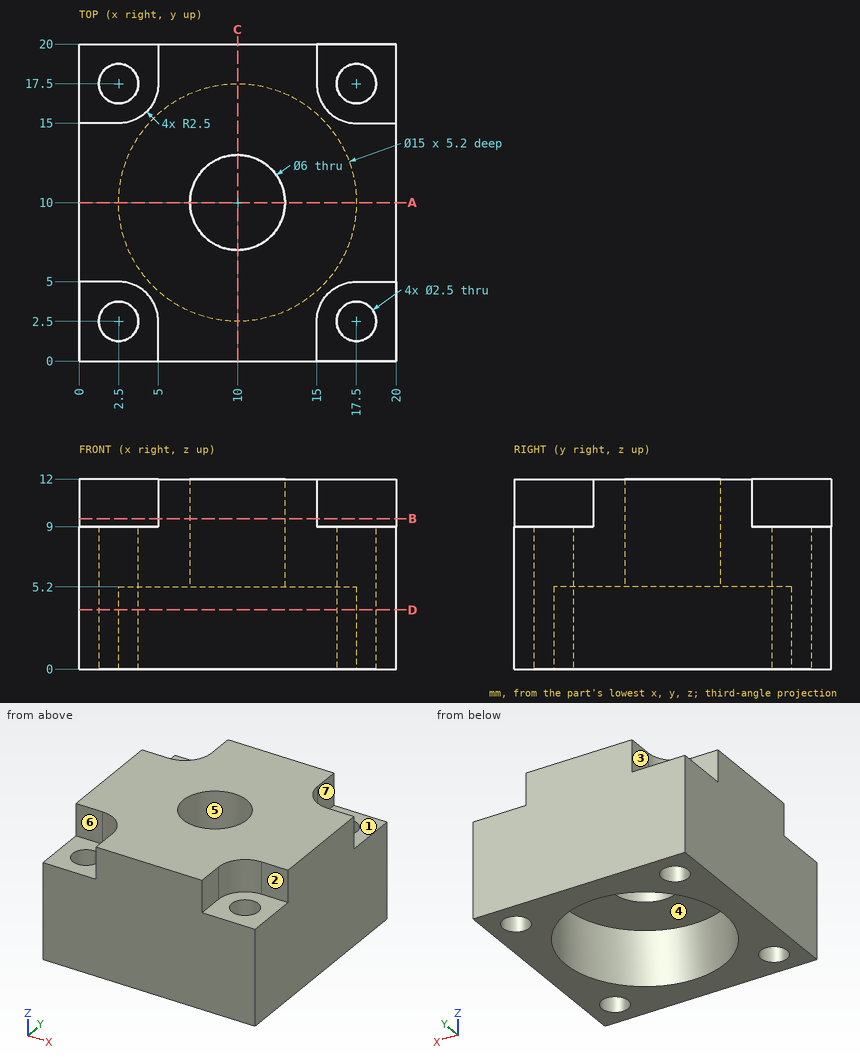
Here's the drawing with two shaded views (mm, measured from the low corner). I have some questions. A direction names the side the tool comes from. Give positions to 0.01 mm unless a question says otherwise; leave off trailing zeros. Loops run counter-clockwise (first coordinate to the right, second up) from the corner with the lowest first, then second, coordinate; pieces in that order, holes last. Notation, with made-up numbers: (69.25, 52) -> (104.25, 52) arc R17 ccw to (104.25, 65) -> close; hole circle Ø6 at (1, -30.5). An arc over 180 degrees is marked (long way). Use one line per item in the form item = value.
1) If we section it at A-A (y = 10): Please give me the cut outline in (x, z), plus the area to 3 significant figures.
Answers:
outline = (0, 0) -> (2.5, 0) -> (2.5, 5.2) -> (7, 5.2) -> (7, 12) -> (0, 12) -> close; (13, 5.2) -> (17.5, 5.2) -> (17.5, 0) -> (20, 0) -> (20, 12) -> (13, 12) -> close
area = 121 mm²
2) If we section it at B-B (z = 9.5): Please give me the cut outline in (x, y).
Answers:
outline = (0, 5) -> (2.5, 5) arc R2.5 cw to (5, 2.5) -> (5, 0) -> (15, 0) -> (15, 2.5) arc R2.5 cw to (17.5, 5) -> (20, 5) -> (20, 15) -> (17.5, 15) arc R2.5 cw to (15, 17.5) -> (15, 20) -> (5, 20) -> (5, 17.5) arc R2.5 cw to (2.5, 15) -> (0, 15) -> close; hole circle Ø6 at (10, 10)
3) Will these pins go through, and if not, where does the flat tip stop? pin 1 (2.5 mm diameter, centred on x = 3, y = 18.5, fed in from +Z); pin 2 (0.8 mm diameter, centred on x = 18, z = 11, fed in from -Y); pin 3 (4.5 mm diameter, centred on x = 12.5, y = 9, fed in from -Z).
Answers:
pin_1 = 9
pin_2 = 5
pin_3 = 5.2
4) If we section it at D-D (z = 3.75): Please give me the cut outline in (x, y).
Answers:
outline = (0, 0) -> (20, 0) -> (20, 20) -> (0, 20) -> close; hole circle Ø2.5 at (2.5, 2.5); hole circle Ø2.5 at (2.5, 17.5); hole circle Ø15 at (10, 10); hole circle Ø2.5 at (17.5, 2.5); hole circle Ø2.5 at (17.5, 17.5)
5) For the marked faces 1, 2, 3 and 4, which set-ups out of +Z, -Z, +X, -X, +Y, -Y let a thin tool reach every point of the face, with its end or its side?
Answers:
face_1 = +Z, +X, +Y
face_2 = +Z, +X, -Y
face_3 = +Z, -X, +Y
face_4 = -Z
6) We'd pull the mould along Y, two halves only. Please class the marked faces 5, 6 and 7: released by +Y, released by -Y, zero draft, split by the parting line, or undercut.
Answers:
face_5 = undercut
face_6 = released by -Y
face_7 = zero draft
7) I need wall thicknesses on line 1 along X through (y, z) = (2.5, 5.75); line 2 along Y through (x, z) = (10, 2.2). Which ranges of each line are inside material? Lowest first, please.
Answers:
line_1 = 0 to 1.25, 3.75 to 16.25, 18.75 to 20
line_2 = 0 to 2.5, 17.5 to 20
